from build123d import *

# Parameters (mm, degrees)
BOSS_EXTRUDE1_DEPTH = 1


with BuildPart() as part:
    # Sketch1 → Revolve1 (revolve)
    with BuildSketch(Plane.XY):
        with BuildLine():
            Line((8.06, -0.352610192), (8.06, -1.359072581))
            Line((8.06, -1.359072581), (6.3, -1.359072581))
            Line((6.3, -1.359072581), (6.3, 2.140927419))
            Line((6.3, 2.140927419), (8.06, 2.140927419))
            Line((8.06, 2.140927419), (8.06, 1.13446503))
            ThreePointArc((8.06, 1.13446503), (8.803537611, 0.390927419), (8.06, -0.352610192))
        make_face()
    revolve(axis=Axis((0, -133.995441592, 0), (0, 1, 0)))

    # Sketch2 → Boss-Extrude1 (add)
    with BuildSketch(Plane(origin=(0, 2.140927419, 0), x_dir=(1, 0, 0), z_dir=(0, 1, 0))):
        with BuildLine():
            Line((6.298583041, 0.133610171), (8.059984934, -0.015584327))
            ThreePointArc((8.059984934, -0.015584327), (8.054947739, 0.285336502), (8.038679535, 0.585859486))
            Line((8.038679535, 0.585859486), (6.281305641, 0.484973654))
            ThreePointArc((6.281305641, 0.484973654), (6.292397308, 0.309412531), (6.298583041, 0.133610171))
        make_face()
    extrude(amount=BOSS_EXTRUDE1_DEPTH)


solid = part.part
Build history of the part. All positions in model axes, mm. A direction names the side the tool comes from. Round coordinates to 2 decimals unless told otherwise and drop trailing zeros. Loops run counter-clockwise (first coordinate to the right, second up) from the corner with the lowest first, then second, coordinate; pieces in that order, holes last. Notation, with made-up numbers: (-13.75, 0.25) -> (27.25, 0.25) arc R18 cw to (27.25, 34.25) -> close; hole circle Ø6 at (-36.75, 30.5). An arc over 180 degrees is marked (long way). Answer in a Markdown table with one row per item.
Item 1: Drill centre lines: L1, parallel to X at y = -0.55, z = 0; L2, parallel to Y at x = -5.5, z = 4. Where is each one in solid material? Low to high. Write a range as [from, to].
Answers below:
| item | result |
|---|---|
| L1 | x = [-8.06, -6.3], [6.3, 8.06] |
| L2 | y = [-1.36, 2.14] |
Item 2: Saw through at A-A (x = 0). Write the cut outline in (y, z).
Answers below:
| item | result |
|---|---|
| outline | (-1.36, -8.06) -> (-0.35, -8.06) arc R0.74 ccw to (1.13, -8.06) -> (2.14, -8.06) -> (2.14, -6.3) -> (-1.36, -6.3) -> close; (-1.36, 6.3) -> (2.14, 6.3) -> (2.14, 8.06) -> (1.13, 8.06) arc R0.74 ccw to (-0.35, 8.06) -> (-1.36, 8.06) -> close |
Item 3: Saw through at B-B (y = 1.8). Write the cut outline in (x, z).
Answers below:
| item | result |
|---|---|
| outline | circle Ø16.12 at (0, 0); hole circle Ø12.6 at (0, 0) |
Item 4: Which spindle directions (+Z, -Z, +X, -X, +Y, -Y) get a long thin tool onto all of the face, cutting with end or side? Do faces 1 (the flat face through (7.172, 2.634, -0.536)), 2 (the cylindrical face through (-6.4, -0.9, 4.9)), 3 (the flat face through (7.17, 2.63, -0.06)). Say none if no direction does.
Answers below:
| item | result |
|---|---|
| face 1 | -Z, -X, +Y |
| face 2 | -Y |
| face 3 | +Z, -X, +Y |
Item 5: Pin check, flat tips, straight feed: pin 1 (10 mm diameter, centred on x = 3, z = -5.5, fed in from +Y); pin 2 (2 mm diameter, centred on y = 0.5, z = -6.5, fed in from +X). Stop position of each tip, or through.
Answers below:
| item | result |
|---|---|
| pin 1 | stops at y = 2.14 |
| pin 2 | stops at x = 6.87 |
